Autodesk Inventor part; units mm, degrees
ref_plane "YZ Plane" through (0, 0, 0) normal (1, 0, 0) x (0, 1, 0)
ref_plane "XZ Plane" through (0, 0, 0) normal (0, 1, 0) x (-1, 0, 0)
ref_plane "XY Plane" through (0, 0, 0) normal (0, 0, 1) x (1, 0, 0)
sketch "Sketch1" plane through (0, 0, 0) normal (0, 0, 1) x (1, 0, 0)
  line L0 (-15.5, 12) -> (15.5, 12)
  line L1 (15.5, 12) -> (15.5, -12)
  line L2 (15.5, -12) -> (-15.5, -12)
  line L3 (-15.5, -12) -> (-15.5, 12)
  line L4 (-15.5, 12) -> (15.5, -12) construction
  line L5 (15.5, 12) -> (-15.5, -12) construction
  point P0 (0, 0)
  dimension "d0" = 24
  dimension "d1" = 31
extrude "Extrusion1" add sketch "Sketch1" along normal blind 3
fillet "Fillet1" radius 0.5 4 edges at (15.5, 12, 1.5) (15.5, -12, 1.5) (-15.5, -12, 1.5) (-15.5, 12, 1.5)
sketch "Sketch4" plane through (0, 0, 3) normal (0, 0, 1) x (1, 0, 0)
  line L0 (-7, -10) -> (7, -10)
  line L1 (13, -4) -> (13, 4)
  line L2 (7, 10) -> (-7, 10)
  line L3 (-13, 4) -> (-13, -4)
  line L4 (-13, -10) -> (13, 10) construction
  line L5 (13, -10) -> (-13, 10) construction
  arc A0 (-13, -4) -> (-7, -10) centre (-7, -4) ccw
  arc A1 (7, -10) -> (13, -4) centre (7, -4) ccw
  line L6 (-7, 10) -> (-13, 4)
  line L7 (13, 4) -> (7, 10)
  point P0 (0, 0)
  point P1 (0, 0)
  dimension "d13" = 20
  dimension "d14" = 26
  dimension "d41" = 6
  dimension "d42" = 6
  dimension "d43" = 6
  dimension "d44" = 6
  dimension "d45" = 6
extrude "Extrusion4" add sketch "Sketch4" along normal blind 17
sketch "Sketch8" plane through (0, 0, 0) normal (0, 1, 0) x (-1, 0, 0)
  line L0 (-13, 10) -> (-14, 5)
  line L1 (-14, 5) -> (-13, 5)
  line L2 (-15, 3) -> (15, 3)
  line L3 (-13, 5) -> (-13, 10)
  line L4 (-13, 3) -> (-13, 20)
  point P0 (0, 0)
  dimension "d36" = 2
  dimension "d37" = 1
  dimension "d38" = 5
extrude "Extrusion7" add sketch "Sketch8" along normal mid plane 7
mirror "Mirror1" about plane through (0, 0, 0) normal (1, 0, 0) of "Extrusion7"
sketch "Sketch5" plane through (0, 0, 0) normal (0, 0, -1) x (-1, 0, 0)
  line L0 (-7.5, 8.5) -> (7.5, 8.5)
  line L1 (12.5, 3.5) -> (12.5, -4.5)
  line L2 (8.5, -8.5) -> (-8.5, -8.5)
  line L3 (-12.5, -4.5) -> (-12.5, 3.5)
  line L4 (-12.5, 8.5) -> (12.5, -8.5) construction
  line L5 (12.5, 8.5) -> (-12.5, -8.5) construction
  line L6 (-12.5, 3.5) -> (-7.5, 8.5)
  line L7 (7.5, 8.5) -> (12.5, 3.5)
  arc A0 (-12.5, -4.5) -> (-8.5, -8.5) centre (-8.5, -4.5) ccw
  arc A1 (8.5, -8.5) -> (12.5, -4.5) centre (8.5, -4.5) ccw
  point P0 (0, 0)
  dimension "d18" = 17
  dimension "d19" = 25
  dimension "d20" = 5
  dimension "d21" = 5
  dimension "d22" = 5
  dimension "d23" = 5
  dimension "d24" = 4
extrude "Extrusion5" cut sketch "Sketch5" against normal blind 17
sketch "Sketch7" plane through (0, 0, 17) normal (0, 0, -1) x (-1, 0, 0)
  line L0 (0.5, 3.7551) -> (-0.5, 3.7551)
  line L1 (-0.5, 3.7551) -> (-0.5, 0.5551)
  line L2 (-0.5, 0.5551) -> (0.5, 0.5551)
  line L3 (0.5, 0.5551) -> (0.5, 3.7551)
  line L4 (0.5, 3.7551) -> (-0.5, 0.5551) construction
  line L5 (-0.5, 3.7551) -> (0.5, 0.5551) construction
  line L6 (7.6155, -0.4449) -> (6.6155, -0.4449)
  line L7 (6.6155, -0.4449) -> (6.6155, -3.6449)
  line L8 (6.6155, -3.6449) -> (7.6155, -3.6449)
  line L9 (7.6155, -3.6449) -> (7.6155, -0.4449)
  line L10 (7.6155, -0.4449) -> (6.6155, -3.6449) construction
  line L11 (6.6155, -0.4449) -> (7.6155, -3.6449) construction
  line L12 (0, 0) -> (0, -2.165)
  line L13 (-7.6155, -0.4449) -> (-6.6155, -0.4449)
  line L14 (-6.6155, -0.4449) -> (-6.6155, -3.6449)
  line L15 (-6.6155, -3.6449) -> (-7.6155, -3.6449)
  line L16 (-7.6155, -3.6449) -> (-7.6155, -0.4449)
  line L17 (-7.6155, -0.4449) -> (-6.6155, -3.6449) construction
  line L18 (-6.6155, -0.4449) -> (-7.6155, -3.6449) construction
  point P0 (0, 2.1551)
  point P1 (7.1155, -2.0449)
  point P2 (-7.1155, -2.0449)
  point P3 (-7.1155, -0.4449)
  dimension "d27" = 1
  dimension "d28" = 1
  dimension "d29" = 3.2
  dimension "d30" = 3.2
  dimension "d35" = 1
extrude "Extrusion6" add sketch "Sketch7" along normal blind 14
equation "\"d21\" = d20"
equation "\"d22\" = d20"
equation "\"d23\" = d22"
properties part number "power_socket_24V_2" material "ABS Plastic"
Input: part model. Units: mm. Frame: model coordinates. A direction names the side the tool comes from. Coordinates: 2 decimals unless noted, no trailing zeros. Order: outer loops, then holes, each group sorted by start corner. A loop starts at its lowest first (then second) coordinate and runs counter-clockwise, first axis right, second up. Notation, with made-up numbers: M 71.25,55.5 L 111.25,55.5 A23 cw 111.25,81.5 Z; hole C -28.75,31 d6. An arc over 180 degrees is marked long. Answer as CSV lines item,"result".
1. Material intervals for line 1 (Y direction, x = -7, z = 3.25); line 2 (Y direction, x = 8.5, z = 2); line 3 (Y direction, x = 4.5, z = 1), sorted ascending. Write a range as from..to.
Reported:
line 1,"-10..-8.5, -3.64..-0.44, 8.5..10"
line 2,"-12..-8.5, 7.5..12"
line 3,"-12..-8.5, 8.5..12"
2. Pull-direction query (Y, two-part tool) for faces 1 (the flat face through (13.3, -3.5, 6.4)), 2 (the flat face through (10, 7, 11)), 3 (the flat face through (0, 0.555, 10)), 4 (the flat face through (-7, -2, 3)); classes: released by +Y, released by -Y, zero draft, split by the parting line, or undercut.
Reported:
face 1,"released by -Y"
face 2,"released by +Y"
face 3,"undercut"
face 4,"undercut"
3. Section B-B (z = 2). Return the cut outline in (x, y), then the cut area to 3 significant figures.
Reported:
outline,"M -15.5,-11.5 A0.5 ccw -15,-12 L 15,-12 A0.5 ccw 15.5,-11.5 L 15.5,11.5 A0.5 ccw 15,12 L -15,12 A0.5 ccw -15.5,11.5 Z; hole M -12.5,-4.5 A4 ccw -8.5,-8.5 L 8.5,-8.5 A4 ccw 12.5,-4.5 L 12.5,3.5 L 7.5,8.5 L -7.5,8.5 L -12.5,3.5 Z"
area,"351 mm2"
4. Section A-A (z = 10.75). Return the cut outline in (x, y).
Reported:
outline,"M -13,-4 A6 ccw -7,-10 L 7,-10 A6 ccw 13,-4 L 13,4 L 7,10 L -7,10 L -13,4 Z; M -7.62,-3.64 L -6.62,-3.64 L -6.62,-0.44 L -7.62,-0.44 Z; M -0.5,0.56 L 0.5,0.56 L 0.5,3.76 L -0.5,3.76 Z; M 6.62,-3.64 L 7.62,-3.64 L 7.62,-0.44 L 6.62,-0.44 Z; hole M -12.5,-4.5 A4 ccw -8.5,-8.5 L 8.5,-8.5 A4 ccw 12.5,-4.5 L 12.5,3.5 L 7.5,8.5 L -7.5,8.5 L -12.5,3.5 Z"
5. Section D-D (y = 4.5). Return the cut outline in (x, z), then the cut area to 3 significant figures.
Reported:
outline,"M -15.5,0 L -11.5,0 L -11.5,17 L 11.5,17 L 11.5,0 L 15.5,0 L 15.5,3 L 12.5,3 L 12.5,20 L -12.5,20 L -12.5,3 L -15.5,3 Z"
area,"127 mm2"
6. Section C-C (x = 0). Return the cut outline in (y, z), then the cut area to 3 significant figures.
Reported:
outline,"M -12,0 L -8.5,0 L -8.5,17 L 0.56,17 L 0.56,3 L 3.76,3 L 3.76,17 L 8.5,17 L 8.5,0 L 12,0 L 12,3 L 10,3 L 10,20 L -10,20 L -10,3 L -12,3 Z"
area,"168 mm2"
7. First-contact query: P1, Ø2, axis at x = 5, y = -6.5, coming from the -Z side; P2, Ø5, axis at x = -3, y = 6.5, coming from the -Z side; P3, Ø1, axis at y = -2.5, z = 8, coming from the -X side; P4, Ø0.5, axis at x = 7, z = 8, coming from the -Y side. Flat tips, straight axial feed; report the tip coordinate or a pass-through.
Reported:
P1,"z = 17"
P2,"z = 0"
P3,"x = -13.5"
P4,"y = -10"
8. Access query for faces 5 (the flat face through (10, 6, 8)), 6 (the flat face through (-13.5, 0, 5)), 7 (the flat face through (0, -12, 1)). Directions: +Z, -Z, +X, -X, +Y, -Y. A direction counts if a zero-diameter tool reaches every point of the face in a straight line with its end or side. Return the directions, or none.
Reported:
face 5,"-Z"
face 6,"-X, +Y, -Y"
face 7,"+Z, -Z, +X, -X, -Y"
